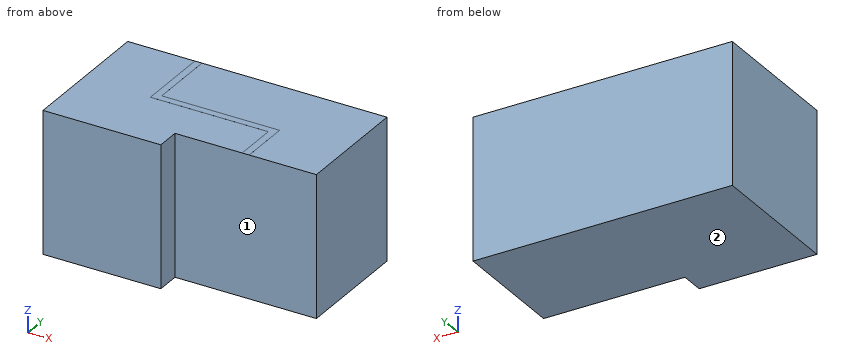
Autodesk Inventor part; units mm, degrees
ref_plane "YZ Plane" through (0, 0, 0) normal (1, 0, 0) x (0, 1, 0)
ref_plane "XZ Plane" through (0, 0, 0) normal (0, 1, 0) x (-1, 0, 0)
ref_plane "XY Plane" through (0, 0, 0) normal (0, 0, 1) x (1, 0, 0)
sketch "スケッチ1" plane through (0, 0, 0) normal (0, 0, 1) x (1, 0, 0)
  line L0 (0, 0) -> (0, 600)
  line L1 (0, 600) -> (1100, 600)
  line L2 (1100, 600) -> (1100, 100)
  line L3 (1100, 100) -> (500, 100)
  line L4 (500, 100) -> (500, 0)
  line L5 (500, 0) -> (0, 0)
  line L6 (285, 600) -> (315, 600)
  line L7 (315, 600) -> (315, 285)
  line L8 (315, 285) -> (285, 285)
  line L9 (285, 285) -> (285, 600)
  line L10 (285, 285) -> (815, 285)
  line L11 (815, 285) -> (815, 315)
  line L12 (815, 315) -> (285, 315)
  line L13 (285, 315) -> (285, 285)
  line L14 (785, 100) -> (815, 100)
  line L15 (815, 100) -> (815, 315)
  line L16 (815, 315) -> (785, 315)
  line L17 (785, 315) -> (785, 100)
  point P0 (285, 300)
  point P1 (0, 300)
  point P2 (800, 100)
  point P3 (800, 100)
  dimension "d0" = 600
  dimension "d1" = 1100
  dimension "d2" = 500
  dimension "d3" = 600
  dimension "d4" = 100
  dimension "d5" = 30
  dimension "d6" = 285
extrude "押し出し1" add sketch "スケッチ1" along normal blind 600 contours L0 L1 L9 L8 L10 L17 L3 L4 L5 | L1 L2 L3 L15 L11 L12 L7
sketch "スケッチ2" plane through (0, 0, 0) normal (0, 0, -1) x (-1, 0, 0)
  line L0 (-285, 285) -> (-785, 285)
  line L1 (-785, 285) -> (-785, 100)
  line L2 (-285, 600) -> (-285, 285)
  line L3 (-815, 315) -> (-315, 315)
  line L4 (-315, 315) -> (-315, 600)
  line L5 (-1100, 600) -> (-315, 600)
  line L6 (-1100, 100) -> (-1100, 600)
  line L7 (-815, 100) -> (-1100, 100)
  line L8 (-815, 100) -> (-815, 315)
  line L9 (-285, 600) -> (-315, 600)
  line L10 (-785, 100) -> (-815, 100)
extrude "押し出し2" add sketch "スケッチ2" against normal blind 600.1 contours L0 L1 L10 L8 L3 L4 L9 L2
sketch "スケッチ3" plane through (0, 0, 600.1) normal (0, 0, 1) x (1, 0, 0)
  line L0 (285, 600) -> (285, 285)
  line L1 (285, 285) -> (785, 285)
  line L2 (815, 100) -> (815, 315)
  line L3 (815, 315) -> (315, 315)
  point P0 (0, 0)
  point P1 (800, 300)
  point P2 (300, 300)
  point P3 (300, 500)
  point P4 (600, 298.5149)
  dimension "d11" = 15
  dimension "d12" = 15
  dimension "d13" = 15
  dimension "d14" = 15
  dimension "d15" = 200
  dimension "d16" = 200
properties part number "River 2_赤"
Read the model definition and answer for the solid it produces. Units are mm, in the model's axes. Face numbers are marked on the shaded views. A direction names the side the tool comes from. Give positions to 0.01 mm unless a question says otherwise; leave off trailing zeros. Write each loop counter-clockwise with the first axis right and the second up, starting at its lowest first coordinate (ties: lowest second). Pieces come first, ordered by that corner, then holes. Notation, with made-up numbers: (57, 26) -> (72, 26) arc R14 cw to (72, 49) -> close; hole circle Ø7 at (-37, -21). An arc over 180 degrees is marked (long way). Answer as a JSON object with one key per item and string values. Group by question number.
1) Consider L1, parallel to Y at x = 816.5, z = 456; L2, parallel to Z at x = 151, y = 362; L3, parallel to X at y = 89.5, z = 557.5. Determine where each line is inside the solid, lowest interval first. Write a range as from..to.
2) Each of these flat-tipped pins is pushed along its axis until it touches: P1, Ø10, axis at x = 432.5, y = 294, coming from the -Z side; P2, Ø2, axis at x = 737, z = 460.5, coming from the -Y side; P3, Ø3, axis at x = 758, y = 481, coming from the +Z side; P4, Ø1, axis at y = 93, z = 460.5, coming from the +X side. Where does it stop, or does it pass through?
3) A tool of negligible diameter and unlimited length cuts with its end or side. For the marked faces 1 and 2, from which of +Z, -Z, +X, -X, +Y, -Y can it reach the whole face along a straight path? Write none if from no direction.
4) Find section A-A (x = 516). Write down the section's boundary in (y, z).
5) Find section B-B (z = 93). Write down the section's boundary in (x, y).
6) Find section C-C (y = 70). Write down the section's boundary in (x, z).
Values follow:
{
 "1": {"L1": "y = 100..600", "L2": "z = 0..600", "L3": "x = 0..500"},
 "2": {"P1": "stops at z = 0", "P2": "stops at y = 100", "P3": "stops at z = 600", "P4": "stops at x = 500"},
 "3": {"face 1": "+Z, -Z, +X, -Y", "face 2": "-Z, +X, -X, +Y, -Y"},
 "4": {"outline": "(100, 0) -> (600, 0) -> (600, 600) -> (315, 600) -> (315, 600.1) -> (285, 600.1) -> (285, 600) -> (100, 600) -> close"},
 "5": {"outline": "(0, 0) -> (500, 0) -> (500, 100) -> (1100, 100) -> (1100, 600) -> (0, 600) -> close"},
 "6": {"outline": "(0, 0) -> (500, 0) -> (500, 600) -> (0, 600) -> close"}
}
